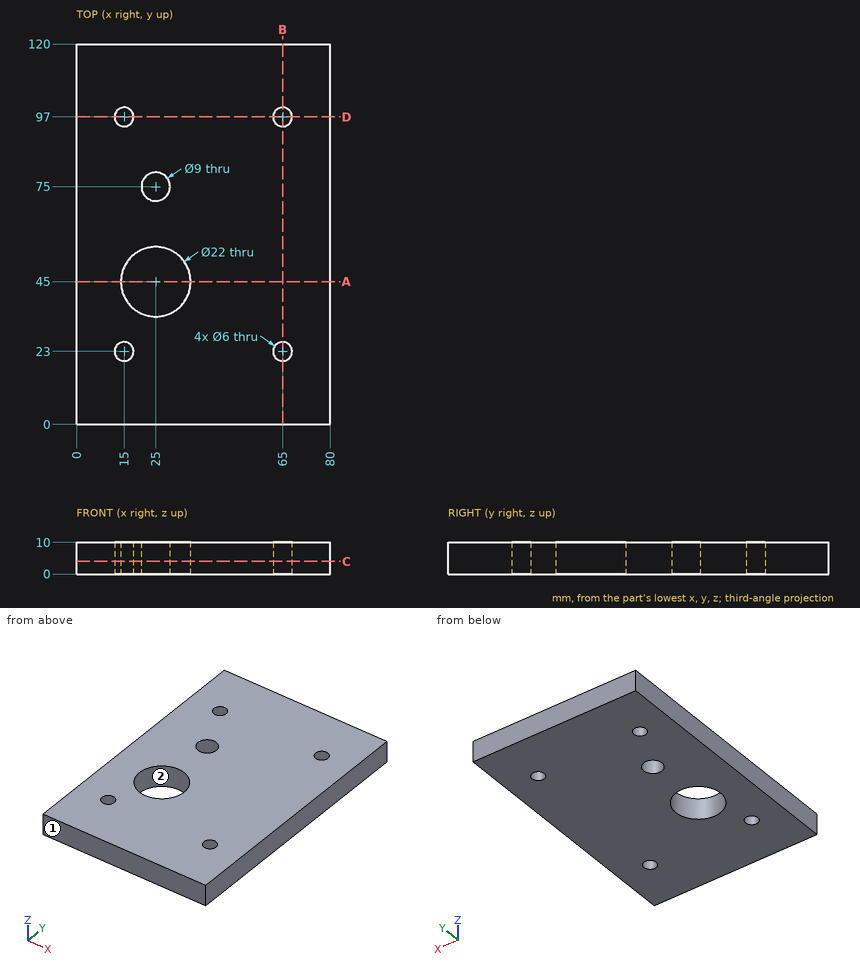
Check sheet for the drawn part. Datum: minimum x, y, z corner. Units: mm. Coordinates: 2 decimals unless noted, no trailing zeros. Loops run counter-clockwise (first coordinate to the right, second up) from the corner with the lowest first, then second, coordinate; pieces in that order, holes last. Notation, with made-up numbers: (85, -10.75) -> (141, -10.75) arc R17 ccw to (141, 20.25) -> close; hole circle Ø5 at (-2, 48). An arc over 180 degrees is marked (long way). Answer in a Markdown table with one row per item.
1. Sectioned sample at D-D, the plane y = 97. Record the boundary of the cut face in (x, z), then the cut area to 3 significant figures.
Check values:
| item | result |
|---|---|
| outline | (0, 0) -> (12, 0) -> (12, 10) -> (0, 10) -> close; (18, 0) -> (62, 0) -> (62, 10) -> (18, 10) -> close; (68, 0) -> (80, 0) -> (80, 10) -> (68, 10) -> close |
| area | 680 mm2 |
2. Sectioned sample at A-A, the plane y = 45. Record the boundary of the cut face in (x, z).
Check values:
| item | result |
|---|---|
| outline | (0, 0) -> (14, 0) -> (14, 10) -> (0, 10) -> close; (36, 0) -> (80, 0) -> (80, 10) -> (36, 10) -> close |
3. Material ranges on line 1 along Y through (x, z) = (65, 5.25); line 2 along Y through (x, z) = (63, 8); line 3 along X through (y, z) = (23.5, 8), recorded low to high. Write a range as [from, to].
Check values:
| item | result |
|---|---|
| line 1 | y = [0, 20], [26, 94], [100, 120] |
| line 2 | y = [0, 20.76], [25.24, 94.76], [99.24, 120] |
| line 3 | x = [0, 12.04], [17.96, 62.04], [67.96, 80] |
4. Release check for a two-part mould opening along X. For the marked faces 1 and 2 record: released by +X, released by -X, zero draft, split by the parting line, or undercut.
Check values:
| item | result |
|---|---|
| face 1 | zero draft |
| face 2 | undercut |
5. Sectioned sample at C-C, the plane z = 4. Record the boundary of the cut face in (x, y), then the cut area to 3 significant figures.
Check values:
| item | result |
|---|---|
| outline | (0, 0) -> (80, 0) -> (80, 120) -> (0, 120) -> close; hole circle Ø6 at (15, 23); hole circle Ø6 at (15, 97); hole circle Ø22 at (25, 45); hole circle Ø9 at (25, 75); hole circle Ø6 at (65, 23); hole circle Ø6 at (65, 97) |
| area | 9,040 mm2 |
6. Sectioned sample at B-B, the plane x = 65. Record the boundary of the cut face in (y, z).
Check values:
| item | result |
|---|---|
| outline | (0, 0) -> (20, 0) -> (20, 10) -> (0, 10) -> close; (26, 0) -> (94, 0) -> (94, 10) -> (26, 10) -> close; (100, 0) -> (120, 0) -> (120, 10) -> (100, 10) -> close |
